Work out the finished part from the listing and answer in its coordinate system (mm). Face numbers are marked on the shaded views. A direction names the side the tool comes from. Give positions to 0.01 mm unless a question says otherwise; leave off trailing zeros. Write each loop counter-clockwise with the first axis right and the second up, starting at its lowest first coordinate (ties: lowest second). Pieces come first, ordered by that corner, then holes. Notation, with made-up numbers: (80.25, -3.75) -> (114.25, -3.75) arc R17 ccw to (114.25, 2.25) -> close; hole circle Ø6 at (9, -40). An arc over 180 degrees is marked (long way). Use a Markdown table: item, result. Add a question column.
Q1. Section B-B, the plane x = 1100 is taken. Give the vertices of the cut face in (y, z).
Q2. Section A-A, the plane y = 0 is taken. Give the vertices of the cut face in (x, z).
Q3. Section C-C, the plane x = 0 is taken. Give the vertices of the cut face in (y, z), plus the area to 3 significant figures.
Q4. For the marked faces 4, 5 and 6, determine the directions among +Z, -Z, +X, -X, +Y, -Y from which every point of the face is accessible in a straight line to the end or side of a thin tool.
Q5. Each of these flat-tipped pins is pushed along its axis until it touches: pin 1 Ø6 at (y, z) = (157.5, -65.5) entering from +X; pin 2 Ø5 at (y, z) = (36, -138.5) entering from -X; pin 3 Ø1 at (x, y) = (971, 122.5) entering from -Z. Where does it stop, or does it pass through?
Q6. Section D-D, the plane y = -93 is taken. Give the vertices of the cut face in (x, z), plus the area to 3 significant figures.
Q7. Consider line 1 (Z direction, x = 1100, y = 80); line 2 (Y direction, x = 1041, z = 106); line 3 (X direction, y = 119, z = 200). Determine where each line is inside the solid, lowest interval first.
Q8. For a pull along Z with two mould halves and no side action, classify the marked faces 1, 2 and 3 as pulls with the +Z half, pulls with the -Z half, needs draft (parallel to the pull), parting line crosses it, or undercut.
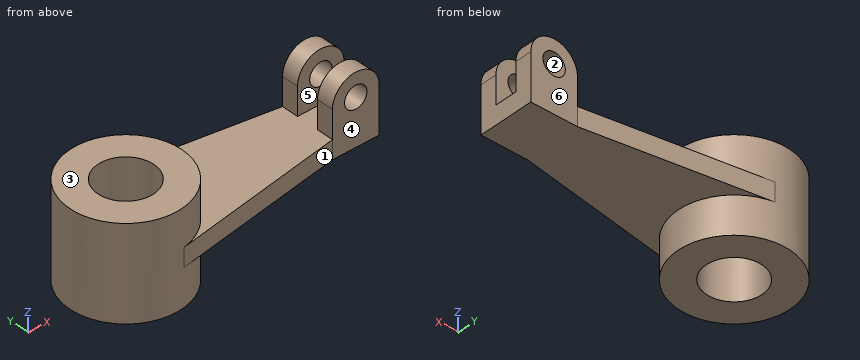
from build123d import *

# Parameters (mm, degrees)
SKETCH1_R           = 300
SKETCH1_R_2         = 150
BOSS_EXTRUDE1_DEPTH = 250
BOSS_EXTRUDE2_DEPTH = 50
SKETCH3_R           = 60
BOSS_EXTRUDE3_DEPTH = 90
SKETCH4_R           = 60
BOSS_EXTRUDE4_DEPTH = 90


with BuildPart() as part:
    # Sketch1 → Boss-Extrude1 (new body, symmetric)
    with BuildSketch(Plane.XY):
        Circle(SKETCH1_R)
        Circle(SKETCH1_R_2, mode=Mode.SUBTRACT)
    extrude(amount=BOSS_EXTRUDE1_DEPTH, both=True)

    # Sketch2 → Boss-Extrude2 (add, symmetric)
    with BuildSketch(Plane.XY):
        with BuildLine():
            Line((46.716887563, 296.340230844), (975, 150))
            Line((975, 150), (1225, 150))
            Line((1225, 150), (1225, -150))
            Line((1225, -150), (975, -150))
            Line((975, -150), (46.716887563, -296.340230844))
            ThreePointArc((46.716887563, -296.340230844), (300, 0), (46.716887563, 296.340230844))
        make_face()
    extrude(amount=BOSS_EXTRUDE2_DEPTH, both=True)

    # Sketch3 → Boss-Extrude3 (add)
    with BuildSketch(Plane.XZ.offset(150)):
        with BuildLine():
            Line((975, 50), (975, 200))
            ThreePointArc((975, 200), (1100, 325), (1225, 200))
            Line((1225, 200), (1225, 50))
            Line((1225, 50), (975, 50))
        make_face()
        with Locations(Location((1100, 200, 0), (0, 0, 270))):  # turned: the seam where the file's is
            Circle(SKETCH3_R, mode=Mode.SUBTRACT)
    extrude(amount=-BOSS_EXTRUDE3_DEPTH)

    # Sketch4 → Boss-Extrude4 (add)
    with BuildSketch(Plane(origin=(0, 150, 0), x_dir=(1, 0, 0), z_dir=(0, 1, 0))):
        with BuildLine():
            Line((975, -200), (975, -50))
            Line((975, -50), (1225, -50))
            Line((1225, -50), (1225, -200))
            ThreePointArc((1225, -200), (1100, -325), (975, -200))
        make_face()
        with Locations(Location((1100, -200, 0), (0, 0, 90))):  # turned: the seam where the file's is
            Circle(SKETCH4_R, mode=Mode.SUBTRACT)
    extrude(amount=-BOSS_EXTRUDE4_DEPTH)


solid = part.part
Result set:
| question | item | result |
|---|---|---|
| 1 | outline | (-150, -50) -> (150, -50) -> (150, 140) -> (60, 140) -> (60, 50) -> (-60, 50) -> (-60, 140) -> (-150, 140) -> close; (-150, 260) -> (-60, 260) -> (-60, 325) -> (-150, 325) -> close; (60, 260) -> (150, 260) -> (150, 325) -> (60, 325) -> close |
| 2 | outline | (-300, -250) -> (-150, -250) -> (-150, 250) -> (-300, 250) -> close; (150, -250) -> (300, -250) -> (300, -50) -> (1225, -50) -> (1225, 50) -> (300, 50) -> (300, 250) -> (150, 250) -> close |
| 3 | outline | (-300, -250) -> (-150, -250) -> (-150, 250) -> (-300, 250) -> close; (150, -250) -> (300, -250) -> (300, 250) -> (150, 250) -> close |
| 3 | area | 150,000 mm2 |
| 4 | face 4 | +Z, -Z, +X, -Y |
| 4 | face 5 | +Z, +X |
| 4 | face 6 | +Z, -Z, +X, +Y |
| 5 | pin 1 | stops at x = 257.16 |
| 5 | pin 2 | stops at x = -298.12 |
| 5 | pin 3 | stops at z = -50 |
| 6 | outline | (-285.22, -250) -> (-117.69, -250) -> (-117.69, 250) -> (-285.22, 250) -> close; (117.69, -250) -> (285.22, -250) -> (285.22, -50) -> (1225, -50) -> (1225, 200) arc R125 ccw to (975, 200) -> (975, 50) -> (285.22, 50) -> (285.22, 250) -> (117.69, 250) -> close; hole circle Ø120 at (1100, 200) |
| 6 | area | 312,000 mm2 |
| 7 | line 1 | z = -50 to 140, 260 to 325 |
| 7 | line 2 | y = -150 to -60, 60 to 150 |
| 7 | line 3 | x = -275.39 to -91.32, 91.32 to 275.39, 975 to 1040, 1160 to 1225 |
| 8 | face 1 | needs draft |
| 8 | face 2 | undercut |
| 8 | face 3 | pulls with the +Z half |
